For this review, use the dimensioned drawing (mm, ordinates from the lowest corner) and the shaded views. A direction names the side the tool comes from. Coordinates: 2 decimals unless noted, no trailing zeros. Order: outer loops, then holes, each group sorted by start corner. A loop starts at its lowest first (then second) coordinate and runs counter-clockwise, first axis right, second up. Notation, with made-up numbers: (52.25, 64.5) -> (94.25, 64.5) arc R35 ccw to (94.25, 98.5) -> close; hole circle Ø1 at (85, -7.5). An arc over 180 degrees is marked (long way). Return JSON: item names as keys, results as strings. Group by question number.
Item 1: Insertion check: pin 1 (6 mm diameter, centred on x = 13.5, z = 7, fed in from -Y); pin 2 (7.5 mm diameter, centred on x = 29.5, z = 10.5, fed in from +Y); pin 3 (4 mm diameter, centred on x = 11.5, z = 2, fed in from +Y) (1 decimal); pin 4 (3 mm diameter, centred on y = 23, z = 4.5, fed in from -X). Each pin has a flat end and moves straight along its axis. Give the tip position at first contact, or say it passes through.
Item 2: Take a section at C-C (x = 30.5). Write out the cut boundary in (y, z).
Item 3: For line 1 along Y through (x, z) = (9.5, 10.5); line 2 along X through (y, z) = (27.5, 6.25); line 3 along X through (y, z) = (10.75, 2.25) (1 decimal), list the stretches that pass through material, from the lowest coordinate up.
Item 4: Take a section at B-B (z = 1). Write out the cut boundary in (x, y) (1 decimal).
Item 5: Take a section at A-A (y = 6). Write out the cut boundary in (x, z) (1 decimal).
Item 6: Draft analysis for pull direction Y (two halves, no side actions). For the marked faces 1, 2, 3 and 4, state which applies: +Y half, -Y half, draft (parallel to the pull), parting line (faces both ways), or undercut.
Item 7: Machinability: for the marked faces 5, 6 and 7, which of the approach directions +Z, -Z, +X, -X, +Y, -Y give a long, thin tool a straight path to every point of the face, cutting with its end or side? Answer none if there is none.
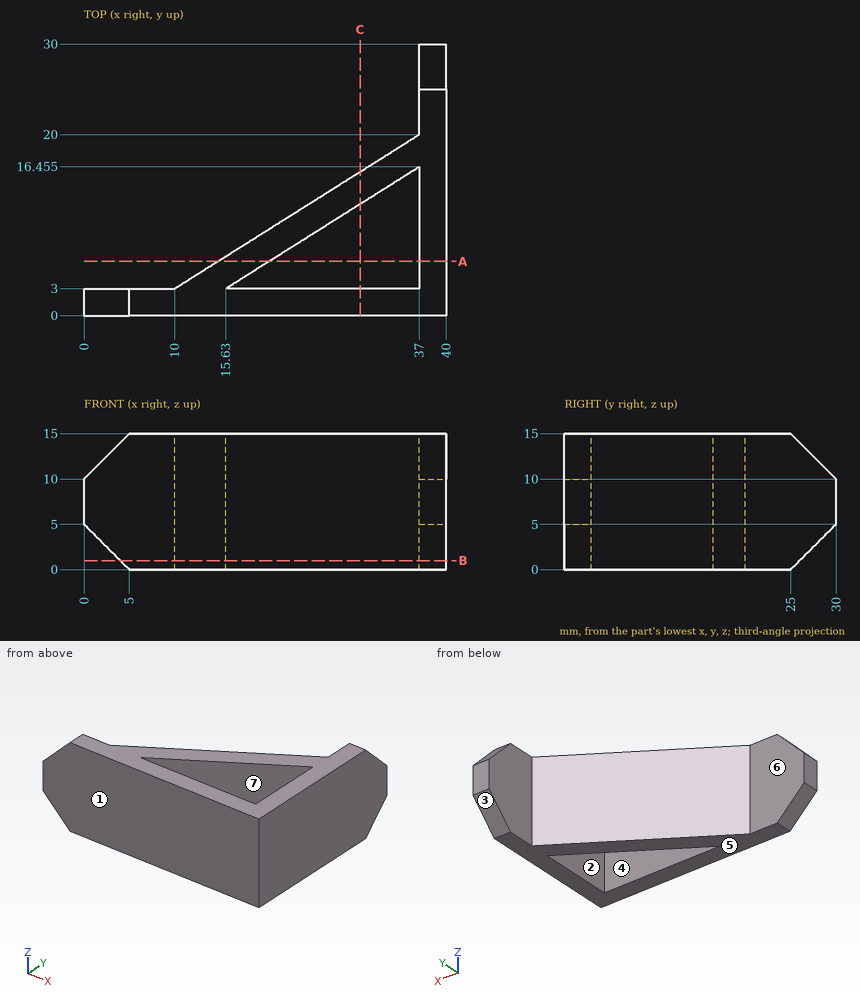
Findings below:
{
 "1": {"pin 1": "stops at y = 0", "pin 2": "stops at y = 17.64", "pin 3": "stops at y = 5.2", "pin 4": "stops at x = 37"},
 "2": {"outline": "(0, 0) -> (3, 0) -> (3, 15) -> (0, 15) -> close; (12.36, 0) -> (15.91, 0) -> (15.91, 15) -> (12.36, 15) -> close"},
 "3": {"line 1": "y = 0 to 3", "line 2": "x = 37 to 40", "line 3": "x = 22.3 to 27.9, 37 to 40"},
 "4": {"outline": "(4, 0) -> (40, 0) -> (40, 26) -> (37, 26) -> (37, 20) -> (10, 3) -> (4, 3) -> close; hole (15.6, 3) -> (37, 3) -> (37, 16.5) -> close"},
 "5": {"outline": "(14.8, 0) -> (20.4, 0) -> (20.4, 15) -> (14.8, 15) -> close; (37, 0) -> (40, 0) -> (40, 15) -> (37, 15) -> close"},
 "6": {"face 1": "-Y half", "face 2": "undercut", "face 3": "+Y half", "face 4": "undercut"},
 "7": {"face 5": "-Z, +X, -X, +Y, -Y", "face 6": "+Z, -Z, -X, +Y", "face 7": "+Z, -Z"}
}
